For this review, take the finished solid that the model builds, in its own axes (mm). Face numbers are marked on the shaded views. Give positions to 0.01 mm unless a question says otherwise; leave off trailing zeros. Order: outer loops, then holes, each group sorted by start corner. A loop starts at its lowest first (then second) coordinate and runs counter-clockwise, first axis right, second up.
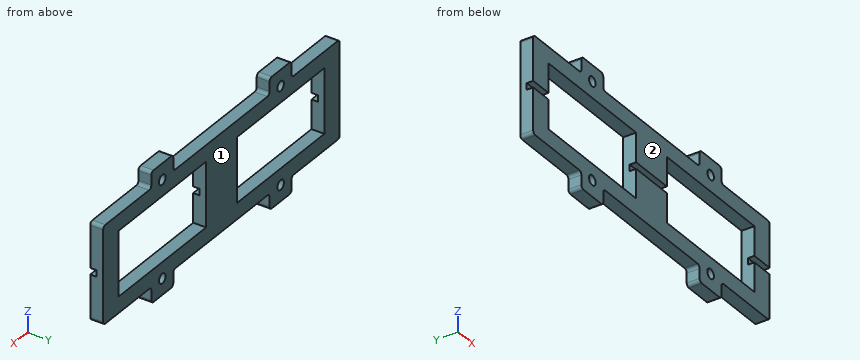
from build123d import *

# Parameters (mm, degrees)
SKETCH_2_W          = 10
SKETCH_2_H          = 5
SKETCH_2_W_2        = 108
SKETCH_2_H_2        = 30
EXTRUDE_1_DEPTH     = 4
SKETCH_3_R          = 1.5
SKETCH_3_W          = 94
SKETCH_3_H          = 20
CUT_EXTRUDE_1_DEPTH = 58.723478759
FILLET_1_R          = 1
SKETCH_4_W          = 14
SKETCH_4_H          = 20
EXTRUDE_2_DEPTH     = 4
SKETCH_6_W          = 7
SKETCH_6_H          = 2
SKETCH_6_W_2        = 14
CUT_EXTRUDE_3_DEPTH = 2


with BuildPart() as part:
    # 草图2 → 凸台-拉伸1 (new body)
    with BuildSketch(Plane(origin=(0, 0, 0), x_dir=(1, 0, 0), z_dir=(0, 1, 0))):
        with Locations((27, 17.5)):
            Rectangle(SKETCH_2_W, SKETCH_2_H)
        with Locations((-27, 17.5)):
            Rectangle(SKETCH_2_W, SKETCH_2_H)
        with Locations((-27, -17.5)):
            Rectangle(SKETCH_2_W, SKETCH_2_H)
        with Locations((27, -17.5)):
            Rectangle(SKETCH_2_W, SKETCH_2_H)
        Rectangle(SKETCH_2_W_2, SKETCH_2_H_2)
    extrude(amount=EXTRUDE_1_DEPTH)

    # 草图3 → 切除-拉伸1 (cut, through all)
    with BuildSketch(Plane.XZ):
        with Locations(Location((-27, 15, 0), (0, 0, 270))):
            Circle(SKETCH_3_R)
        with Locations(Location((27, 15, 0), (0, 0, 90))):
            Circle(SKETCH_3_R)
        with Locations(Location((27, -15, 0), (0, 0, 270))):
            Circle(SKETCH_3_R)
        with Locations(Location((-27, -15, 0), (0, 0, 90))):
            Circle(SKETCH_3_R)
        Rectangle(SKETCH_3_W, SKETCH_3_H)
    extrude(amount=-CUT_EXTRUDE_1_DEPTH, mode=Mode.SUBTRACT)

    # 圆角1
    fillet_1_edges = [part.edges().sort_by_distance(p)[0] for p in [
        (32, 2, -15),
        (54, 2, -15),
        (54, 2, 15),
        (32, 2, 15),
        (32, 2, 20),
        (22, 2, 20),
        (22, 2, 15),
        (-22, 2, 15),
        (-22, 2, 20),
        (-32, 2, 20),
        (-32, 2, 15),
        (-54, 2, 15),
        (-54, 2, -15),
        (-32, 2, -15),
        (-32, 2, -20),
        (-22, 2, -20),
        (-22, 2, -15),
        (22, 2, -15),
        (22, 2, -20),
        (32, 2, -20),
    ]]
    fillet(fillet_1_edges, radius=FILLET_1_R)

    # 草图4 → 凸台-拉伸2 (add)
    with BuildSketch(Plane(origin=(0, 0, 0), x_dir=(1, 0, 0), z_dir=(0, 1, 0))):
        Rectangle(SKETCH_4_W, SKETCH_4_H)
    extrude(amount=EXTRUDE_2_DEPTH)

    # 草图6 → 切除-拉伸3 (cut)
    with BuildSketch(Plane.XZ):
        with Locations((-50.5, 0)):
            Rectangle(SKETCH_6_W, SKETCH_6_H)
        Rectangle(SKETCH_6_W_2, SKETCH_6_H)
        with Locations((50.5, 0)):
            Rectangle(SKETCH_6_W, SKETCH_6_H)
    extrude(amount=-CUT_EXTRUDE_3_DEPTH, mode=Mode.SUBTRACT)


solid = part.part
1) To check wall thickness, follow line 1 (X direction, y = 3.5, z = -3.5); line 2 (Z direction, x = 9, y = 2.35); line 3 (X direction, y = 0.2, z = 17). State the ranges of each line that lie inside material, in increasing order.
Answer sheet:
line 1: x = -54 to -47, -7 to 7, 47 to 54
line 2: z = -15 to -10, 10 to 15
line 3: x = -32 to -22, 22 to 32
2) Clearance check with flat-ended pins moving along their axes: pin 1 (2 mm diameter, centred on x = 37, y = 1, fed in from -Z); pin 2 (1.6 mm diameter, centred on x = 49, y = 0.5, fed in from +Z); pin 3 (1.5 mm diameter, centred on y = 1, z = 15.5, fed in from +X). State where each tip first meets the part, or that it passes through.
Answer sheet:
pin 1: stops at z = -15
pin 2: stops at z = 15
pin 3: stops at x = 53.66
3) We need section D-D on y = 0.65. Count the separate pieces of the cut face and the enclosed holes in it, then the cut area to 3 significant figures.
Answer sheet:
separate pieces: 2
enclosed holes: 4
area: 1,750 mm2
4) We need section C-C on z = 7. Give the boundary of the cut face in (x, y), then the cut area to 3 significant figures.
Answer sheet:
outline: (-54, 0) - (-47, 0) - (-47, 4) - (-54, 4) - close; (-7, 0) - (7, 0) - (7, 4) - (-7, 4) - close; (47, 0) - (54, 0) - (54, 4) - (47, 4) - close
area: 112 mm2
5) Draft analysis for pull direction Y (two halves, no side actions). For the marked faces 1 and 2, state which applies: +Y half, -Y half, draft (parallel to the pull), parting line (faces both ways), or undercut.
Answer sheet:
face 1: +Y half
face 2: -Y half
6) We need section B-B on x = 27. Give the boundary of the cut face in (y, z), then the cut area to 3 significant figures.
Answer sheet:
outline: (0, -20) - (4, -20) - (4, -16.5) - (0, -16.5) - close; (0, -13.5) - (4, -13.5) - (4, -10) - (0, -10) - close; (0, 10) - (4, 10) - (4, 13.5) - (0, 13.5) - close; (0, 16.5) - (4, 16.5) - (4, 20) - (0, 20) - close
area: 56.0 mm2
7) We need section A-A on x = -10.5. Give the boundary of the cut face in (y, z).
Answer sheet:
outline: (0, -15) - (4, -15) - (4, -10) - (0, -10) - close; (0, 10) - (4, 10) - (4, 15) - (0, 15) - close
